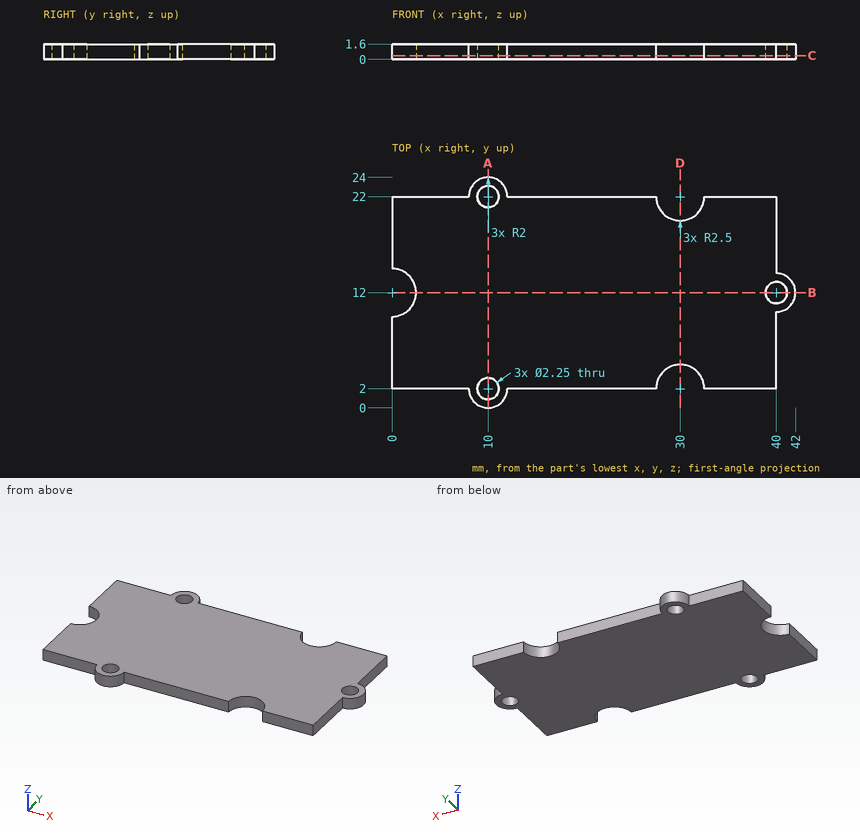
For this review, use the dimensioned drawing (mm, ordinates from the lowest corner) and the shaded views. Round coordinates to 2 decimals unless told otherwise and drop trailing zeros. Write each loop counter-clockwise with the first axis right and the second up, starting at its lowest first coordinate (ties: lowest second). Pieces come first, ordered by that corner, then holes. Notation, with made-up numbers: (-38.75, -27.75) -> (14.25, -27.75) arc R27 cw to (14.25, -7.75) -> close; hole circle Ø9 at (42, 37). An arc over 180 degrees is marked (long way). Use CSV: the item, a comma, the result in double quotes.
(1) Consider section B-B, the plane y = 12. Give the boundary of the cut face in (x, z) (3 decimals), plus the area to 3 significant figures.
Computed values:
outline,"(2.5, 0) -> (38.875, 0) -> (38.875, 1.6) -> (2.5, 1.6) -> close; (41.125, 0) -> (42, 0) -> (42, 1.6) -> (41.125, 1.6) -> close"
area,"59.6 mm²"
(2) Clearance check with flat-ended pins moving along their axes: P1, Ø0.5, axis at x = 35.5, z = 0.5, coming from the +Y side; P2, Ø0.8, axis at x = 5.5, z = 0.5, coming from the -Y side; P3, Ø2, axis at x = 40, y = 12, coming from the -Z side. State where each tip first meets the part, or that it passes through.
Computed values:
P1,"y = 22"
P2,"y = 2"
P3,"through"
(3) Consider section C-C, the plane z = 0.4. Give the boundary of the cut face in (x, y) (3 decimals), plus the area to 3 significant figures.
Computed values:
outline,"(0, 2) -> (8, 2) arc R2 ccw to (12, 2) -> (27.5, 2) arc R2.5 cw to (32.5, 2) -> (40, 2) -> (40, 10) arc R2 ccw to (40, 14) -> (40, 22) -> (32.5, 22) arc R2.5 cw to (27.5, 22) -> (12, 22) arc R2 ccw to (8, 22) -> (0, 22) -> (0, 14.5) arc R2.5 cw to (0, 9.5) -> close; hole circle Ø2.25 at (10, 2); hole circle Ø2.25 at (10, 22); hole circle Ø2.25 at (40, 12)"
area,"777 mm²"
(4) Consider section A-A, the plane x = 10. Give the boundary of the cut face in (y, z) (3 decimals).
Computed values:
outline,"(0, 0) -> (0.875, 0) -> (0.875, 1.6) -> (0, 1.6) -> close; (3.125, 0) -> (20.875, 0) -> (20.875, 1.6) -> (3.125, 1.6) -> close; (23.125, 0) -> (24, 0) -> (24, 1.6) -> (23.125, 1.6) -> close"
(5) To check wall thickness, follow L1, parallel to Y at x = 10, z = 0.85 (3 decimals); L2, parallel to X at y = 12, z = 0.8 (3 decimals); L3, parallel to Y at x = 3, z = 0.5. State the ranges of each line that lie inside material, in increasing order. Write a range as [from, to].
Computed values:
L1,"[0, 0.875], [3.125, 20.875], [23.125, 24]"
L2,"[2.5, 38.875], [41.125, 42]"
L3,"[2, 22]"
(6) Consider section D-D, the plane x = 30. Give the boundary of the cut face in (y, z).
Computed values:
outline,"(4.5, 0) -> (19.5, 0) -> (19.5, 1.6) -> (4.5, 1.6) -> close"
